The listing builds one solid part. Answer for the finished solid, in the listing's coordinates (mm). Face numbers are marked on the shaded views. A direction names the side the tool comes from. Give positions to 0.01 mm unless a question says otherwise; leave off trailing zeros. Write each loop counter-clockwise with the first axis right and the second up, starting at its lowest first coordinate (ties: lowest second). Pieces come first, ordered by that corner, then holes.
```python
from build123d import *

# Parameters (mm, degrees)
SKETCH_W        = 50
SKETCH_H        = 55
PAD_DEPTH       = 20
SKETCH001_W     = 50
SKETCH001_H     = 32
POCKET_DEPTH    = 12
SKETCH002_W     = 32
SKETCH002_H     = 13
POCKET001_DEPTH = 20


with BuildPart() as part:
    # Sketch → Pad (new body)
    with BuildSketch(Plane.XY):
        Rectangle(SKETCH_W, SKETCH_H)
    extrude(amount=PAD_DEPTH)

    # Sketch001 (on Face6 of Pad) → Pocket (cut)
    with BuildSketch(Plane.XY.offset(20)):
        with Locations((0, -8)):
            Rectangle(SKETCH001_W, SKETCH001_H)
    extrude(amount=-POCKET_DEPTH, mode=Mode.SUBTRACT)

    # Sketch002 (on Face5 of Pocket) → Pocket001 (cut)
    with BuildSketch(Plane.XY.offset(20)):
        with Locations((0, 18.5)):
            Rectangle(SKETCH002_W, SKETCH002_H)
    extrude(amount=-POCKET001_DEPTH, mode=Mode.SUBTRACT)


solid = part.part
```
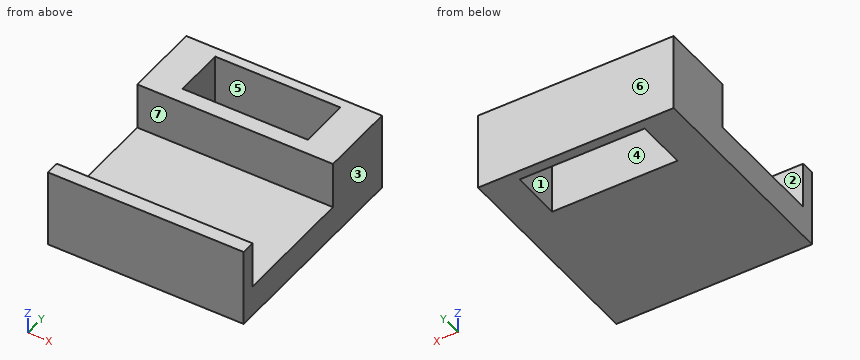
Item 1: A cutting plane is placed at A-A, the plane z = 16.5. Give the vertices of the cut face in (x, y).
Conclusion:
outline: (-25, -27.5) - (25, -27.5) - (25, -24) - (-25, -24) - close; (-25, 8) - (25, 8) - (25, 27.5) - (-25, 27.5) - close; hole (-16, 12) - (16, 12) - (16, 25) - (-16, 25) - close
Item 2: Each of these flat-tipped pins is pushed along its axis until it touches: P1, Ø12, axis at x = -12, y = -14, coming from the -Z side; P2, Ø1, axis at x = 14, y = -2.5, coming from the +Z side. Where does it stop, or does it pass through?
Conclusion:
P1: stops at z = 0
P2: stops at z = 8
Item 3: A cutting plane is placed at B-B, the plane y = 20.5. Give the vertices of the cut face in (x, z), plus the area to 3 significant figures.
Conclusion:
outline: (-25, 0) - (-16, 0) - (-16, 20) - (-25, 20) - close; (16, 0) - (25, 0) - (25, 20) - (16, 20) - close
area: 360 mm2
Item 4: Determine the mould class of the marked faces 1, 2, 3 and 4 for opening direction X: pulls with the +X half, pulls with the -X half, needs draft (parallel to the pull), parting line crosses it, or undercut.
Conclusion:
face 1: undercut
face 2: needs draft
face 3: pulls with the +X half
face 4: undercut
Item 5: Which of the six approach directions +Z, -Z, +X, -X, +Y, -Y give full straight-line access (tool end or side, diameter ignored) to the marked faces 5, 6 and 7?
Conclusion:
face 5: +Z, -Z
face 6: +Z, -Z, +X, -X, +Y
face 7: +Z, +X, -X
Item 6: A cutting plane is placed at D-D, the plane x = -17. Give the vertices of the cut face in (y, z).
Conclusion:
outline: (-27.5, 0) - (27.5, 0) - (27.5, 20) - (8, 20) - (8, 8) - (-24, 8) - (-24, 20) - (-27.5, 20) - close
Item 7: A cutting plane is placed at C-C, the plane x = 0. Give the vertices of the cut face in (y, z), plus the area to 3 significant figures.
Conclusion:
outline: (-27.5, 0) - (12, 0) - (12, 20) - (8, 20) - (8, 8) - (-24, 8) - (-24, 20) - (-27.5, 20) - close; (25, 0) - (27.5, 0) - (27.5, 20) - (25, 20) - close
area: 456 mm2
Item 8: Consider probe 1 along Y at (x, z) = (-1, 15.25); probe 2 along Y at (x, z) = (21, 9.25); probe 3 along X at (y, z) = (19.5, 2). Determine where each line is inside the solid, lowest interval first.
Conclusion:
probe 1: y = -27.5 to -24, 8 to 12, 25 to 27.5
probe 2: y = -27.5 to -24, 8 to 27.5
probe 3: x = -25 to -16, 16 to 25
